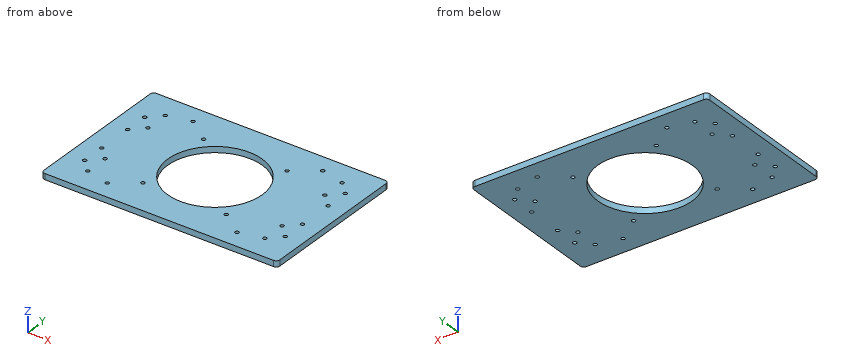
```python
from build123d import *

# Parameters (mm, degrees)
SKETCH_W   = 200
SKETCH_H   = 130
SKETCH_R   = 40
SKETCH_R_2 = 1.5625
PAD_DEPTH  = 5
FILLET_R   = 3


with BuildPart() as part:
    # Sketch → Pad (new body)
    with BuildSketch(Plane.XY):
        with Locations((100, 65)):
            Rectangle(SKETCH_W, SKETCH_H)
        with Locations((100, 65)):
            Circle(SKETCH_R, mode=Mode.SUBTRACT)
        with Locations((45, 115)):
            Circle(SKETCH_R_2, mode=Mode.SUBTRACT)
        with Locations((45, 15)):
            Circle(SKETCH_R_2, mode=Mode.SUBTRACT)
        with Locations((155, 115)):
            Circle(SKETCH_R_2, mode=Mode.SUBTRACT)
        with Locations((155, 15)):
            Circle(SKETCH_R_2, mode=Mode.SUBTRACT)
        with Locations((185, 30)):
            Circle(SKETCH_R_2, mode=Mode.SUBTRACT)
        with Locations((135.353085, 100.338453)):
            Circle(SKETCH_R_2, mode=Mode.SUBTRACT)
        with Locations((64.627773, 29.642413)):
            Circle(SKETCH_R_2, mode=Mode.SUBTRACT)
        with Locations((64.64463, 100.35537)):
            Circle(SKETCH_R_2, mode=Mode.SUBTRACT)
        with Locations((135.352442, 29.63292)):
            Circle(SKETCH_R_2, mode=Mode.SUBTRACT)
        with Locations((175, 20)):
            Circle(SKETCH_R_2, mode=Mode.SUBTRACT)
        with Locations((175, 40)):
            Circle(SKETCH_R_2, mode=Mode.SUBTRACT)
        with Locations((185, 50)):
            Circle(SKETCH_R_2, mode=Mode.SUBTRACT)
        with Locations((175, 90)):
            Circle(SKETCH_R_2, mode=Mode.SUBTRACT)
        with Locations((175, 110)):
            Circle(SKETCH_R_2, mode=Mode.SUBTRACT)
        with Locations((185, 80)):
            Circle(SKETCH_R_2, mode=Mode.SUBTRACT)
        with Locations((185, 100)):
            Circle(SKETCH_R_2, mode=Mode.SUBTRACT)
        with Locations((15, 30)):
            Circle(SKETCH_R_2, mode=Mode.SUBTRACT)
        with Locations((25, 20)):
            Circle(SKETCH_R_2, mode=Mode.SUBTRACT)
        with Locations((25, 40)):
            Circle(SKETCH_R_2, mode=Mode.SUBTRACT)
        with Locations((15, 50)):
            Circle(SKETCH_R_2, mode=Mode.SUBTRACT)
        with Locations((25, 90)):
            Circle(SKETCH_R_2, mode=Mode.SUBTRACT)
        with Locations((25, 110)):
            Circle(SKETCH_R_2, mode=Mode.SUBTRACT)
        with Locations((15, 80)):
            Circle(SKETCH_R_2, mode=Mode.SUBTRACT)
        with Locations((15, 100)):
            Circle(SKETCH_R_2, mode=Mode.SUBTRACT)
    extrude(amount=PAD_DEPTH)

    # Fillet
    fillet_edges = [part.edges().sort_by_distance(p)[0] for p in [
        (0, 0, 2.5),
        (200, 0, 2.5),
        (200, 130, 2.5),
        (0, 130, 2.5),
    ]]
    fillet(fillet_edges, radius=FILLET_R)


solid = part.part
```
Geometry check sheet. Reference: the model listing, model coordinates, mm. Give positions to 0.01 mm unless a question says otherwise; leave off trailing zeros. Order: outer loops, then holes, each group sorted by start corner. A loop starts at its lowest first (then second) coordinate and runs counter-clockwise, first axis right, second up.
1. Section check A-A, the plane x = 87. Enter the section's corners in (y, z), and give its area (3 significant figures).
2. Thickness scan on L1, parallel to Y at x = 25, z = 2.2; L2, parallel to X at y = 110, z = 2.9; L3, parallel to Y at x = 185, z = 2.25. Record the ranges inside material, lowest first.
3. Gauge pin test, flat end, axial feed: pin 1 Ø3.5 at (x, y) = (135.35, 29.63) entering from +Z. Record the tip position at first contact, or that the pin passes through.
4. Section check B-B, the plane z = 1.65. Give the number of separate pieces and of enclosed holes in the cut face, and give its area (3 significant figures).
Values follow:
1. outline: (0, 0) - (27.17, 0) - (27.17, 5) - (0, 5) - close; (102.83, 0) - (130, 0) - (130, 5) - (102.83, 5) - close
1. area: 272 mm2
2. L1: y = 0 to 18.44, 21.56 to 38.44, 41.56 to 88.44, 91.56 to 108.44, 111.56 to 130
2. L2: x = 0 to 23.44, 26.56 to 173.44, 176.56 to 200
2. L3: y = 0 to 28.44, 31.56 to 48.44, 51.56 to 78.44, 81.56 to 98.44, 101.56 to 130
3. pin 1: stops at z = 5
4. separate pieces: 1
4. enclosed holes: 25
4. area: 20,800 mm2
